Check sheet for the modelled part. Datum: model origin and axes. Units: mm. A direction names the side the tool comes from. Give positions to 0.01 mm unless a question says otherwise; leave off trailing zeros. Write each loop counter-clockwise with the first axis right and the second up, starting at its lowest first coordinate (ties: lowest second). Pieces come first, ordered by that corner, then holes. Notation, with made-up numbers: M 66,22 L 122,22 A29 ccw 122,53 Z; hole C 79.25,53.5 d1. An arc over 180 degrees is marked long. Write item = value, one per line. Start each with the question number.
1) Scan lines: L1, parallel to Z at x = 5, y = 7.25; L2, parallel to X at y = 2.5, z = 67; L3, parallel to X at y = 6.25, z = 83.15. Record each from-to range of solid material in increasing order.
2) Sectioned sample at B-B, the plane z = 60. Record the cut outline in (x, y).
3) Sectioned sample at C-C, the plane x = 80.5. Record the cut outline in (y, z), then the cut area to 3 significant figures.
4) Sectioned sample at D-D, the plane z = 110.5. Record the cut outline in (x, y).
5) Draft check along Z on faces 4 (the face through (176.6, 5, 33)), 5 (the face through (0, 9, 74)), 6 (the face through (97, 5, 0)). Enter one of: pulls with the +Z half, pulls with the -Z half, needs draft (parallel to the pull), parting line crosses it, or undercut.
6) Sectioned sample at A-A, the plane x = 5. Record the cut outline in (y, z), then the cut area to 3 significant figures.
7) Gauge pin test, flat ends, axial feed: pin 1 (3 mm diameter, centred on y = 2, z = 91.5, fed in from +X); pin 2 (6 mm diameter, centred on x = 79.5, y = 11, fed in from +Z); pin 3 (22.5 mm diameter, centred on x = 136, z = 127, fed in from +Y). Record the tip position at first contact, or that the pin passes through.
8) Set-up check for faces 1 (the face through (83, 7.5, 75)), 2 (the face through (107, 2.5, 32)), 3 (the face through (107, 4, 62.5)): record each of +Z, -Z, +X, -X, +Y, -Y from which the full face is reachable in a straight line by a thin tool's end or side.
from build123d import *

# Parameters (mm, degrees)
PLATEFRAME_DEPTH          = 150
SKETCH3_R                 = 2.15
HOLESUPPORT_DEPTH         = 7.5
SKETCH4_R                 = 4.15
SKETCH4_R_2               = 2.15
CYLINDRICALSUPPORTS_DEPTH = 12.5
SKETCH8_W                 = 137
SKETCH8_H                 = 60
ITEMLAYOUT_DEPTH          = 5
SKETCH9_W                 = 137
SKETCH9_H                 = 7.5
VELCROHOLES_DEPTH         = 3.5
SKETCH10_W                = 22.1
SKETCH10_H                = 60
OPENHOLE_DEPTH            = 8.5


with BuildPart() as part:
    # Sketch2 → PlateFrame (new body)
    with BuildSketch(Plane.XY):
        Polygon((179.1, 12.5), (191.6, 12.5), (191.6, 5), (184.1, 5), (184.1, 0), (7.5, 0), (7.5, 5), (0, 5), (0, 12.5), (12.5, 12.5), (12.5, 7.5), (179.1, 7.5), align=None)
    extrude(amount=PLATEFRAME_DEPTH)

    # Sketch3 → HoleSupport (cut)
    with BuildSketch(Plane(origin=(0, 12.5, 0), x_dir=(1, 0, 0), z_dir=(0, 1, 0))):
        with Locations((5, -66.85)):
            Circle(SKETCH3_R)
        with Locations((5, -83.15)):
            Circle(SKETCH3_R)
        with Locations((186.6, -66.85)):
            Circle(SKETCH3_R)
        with Locations((186.6, -83.15)):
            Circle(SKETCH3_R)
    extrude(amount=-HOLESUPPORT_DEPTH, mode=Mode.SUBTRACT)

    # Sketch4 → CylindricalSupports (add)
    with BuildSketch(Plane(origin=(0, 12.5, 0), x_dir=(1, 0, 0), z_dir=(0, 1, 0))):
        with Locations((186.6, -66.85)):
            Circle(SKETCH4_R)
        with Locations((186.6, -66.85)):
            Circle(SKETCH4_R_2, mode=Mode.SUBTRACT)
        with Locations((186.6, -83.15)):
            Circle(SKETCH4_R)
        with Locations((186.6, -83.15)):
            Circle(SKETCH4_R_2, mode=Mode.SUBTRACT)
        with Locations((5, -66.85)):
            Circle(SKETCH4_R)
        with Locations((5, -66.85)):
            Circle(SKETCH4_R_2, mode=Mode.SUBTRACT)
        with Locations((5, -83.15)):
            Circle(SKETCH4_R)
        with Locations((5, -83.15)):
            Circle(SKETCH4_R_2, mode=Mode.SUBTRACT)
    extrude(amount=-CYLINDRICALSUPPORTS_DEPTH)

    # Sketch8 → ItemLayout (cut)
    with BuildSketch(Plane(origin=(0, 7.5, 0), x_dir=(1, 0, 0), z_dir=(0, 1, 0))):
        with Locations((108.1, -32.5)):
            Rectangle(SKETCH8_W, SKETCH8_H)
        with Locations((108.1, -117.5)):
            Rectangle(SKETCH8_W, SKETCH8_H)
    extrude(amount=-ITEMLAYOUT_DEPTH, mode=Mode.SUBTRACT)

    # Sketch9 → VelcroHoles (cut, through all)
    with BuildSketch(Plane(origin=(0, 2.5, 0), x_dir=(1, 0, 0), z_dir=(0, 1, 0))):
        with Locations((108.1, -143.75)):
            Rectangle(SKETCH9_W, SKETCH9_H)
        with Locations((108.1, -6.25)):
            Rectangle(SKETCH9_W, SKETCH9_H)
        with Locations((108.1, -91.25)):
            Rectangle(SKETCH9_W, SKETCH9_H)
        with Locations((108.1, -58.75)):
            Rectangle(SKETCH9_W, SKETCH9_H)
    extrude(amount=-VELCROHOLES_DEPTH, mode=Mode.SUBTRACT)

    # Sketch10 → OpenHole (cut, through all)
    with BuildSketch(Plane(origin=(0, 7.5, 0), x_dir=(1, 0, 0), z_dir=(0, 1, 0))):
        with Locations((26.05, -32.5)):
            Rectangle(SKETCH10_W, SKETCH10_H)
    extrude(amount=-OPENHOLE_DEPTH, mode=Mode.SUBTRACT)


solid = part.part
Data:
q1.L1 = 0 to 64.7, 69 to 81, 85.3 to 150
q1.L2 = 0.85 to 2.86, 7.14 to 184.46, 188.74 to 190.75
q1.L3 = 0 to 2.85, 7.15 to 184.45, 188.75 to 191.6
q2.outline = M 0,5 L 7.5,5 L 7.5,0 L 15,0 L 15,7.5 L 12.5,7.5 L 12.5,12.5 L 0,12.5 Z; M 37.1,0 L 39.6,0 L 39.6,7.5 L 37.1,7.5 Z; M 176.6,0 L 184.1,0 L 184.1,5 L 191.6,5 L 191.6,12.5 L 179.1,12.5 L 179.1,7.5 L 176.6,7.5 Z
q3.outline = M 0,0 L 7.5,0 L 7.5,2.5 L 0,2.5 Z; M 0,10 L 2.5,10 L 2.5,55 L 0,55 Z; M 0,62.5 L 7.5,62.5 L 7.5,87.5 L 0,87.5 Z; M 0,95 L 2.5,95 L 2.5,140 L 0,140 Z; M 0,147.5 L 7.5,147.5 L 7.5,150 L 0,150 Z
q3.area = 450 mm2
q4.outline = M 0,5 L 7.5,5 L 7.5,0 L 184.1,0 L 184.1,5 L 191.6,5 L 191.6,12.5 L 179.1,12.5 L 179.1,7.5 L 176.6,7.5 L 176.6,2.5 L 39.6,2.5 L 39.6,7.5 L 12.5,7.5 L 12.5,12.5 L 0,12.5 Z
q5.face_4 = undercut
q5.face_5 = needs draft
q5.face_6 = pulls with the -Z half
q6.outline = M 0,62.7 L 5,62.7 L 5,0 L 12.5,0 L 12.5,64.7 L 0,64.7 Z; M 0,69 L 12.5,69 L 12.5,81 L 0,81 L 0,79 L 5,79 L 5,71 L 0,71 Z; M 0,85.3 L 12.5,85.3 L 12.5,150 L 5,150 L 5,87.3 L 0,87.3 Z
q6.area = 1,100 mm2
q7.pin_1 = 184.1
q7.pin_2 = through
q7.pin_3 = 2.5
q8.face_1 = +Z, -Z, +Y
q8.face_2 = +Y
q8.face_3 = +Y, -Y
